Input: part model. Units: mm. Frame: model coordinates. A direction names the side the tool comes from. Give positions to 0.01 mm unless a question says otherwise; leave off trailing zeros. Loops run counter-clockwise (first coordinate to the right, second up) from the corner with the lowest first, then second, coordinate; pieces in that order, holes last. Notation, with made-up numbers: M -32,9.5 L 10,9.5 A8 cw 10,17.5 Z; hole C 62,-17.75 d8. An arc over 180 degrees is marked long. Use CSV: the item, a comma, the result in double quotes. Start each with the question number.
Q1. Reachability of faces 4 (the flat face through (1.2, 4, 1.2)), 5 (the flat face through (4, 7, -10)), 6 (the flat face through (-5.27, 6.93, 6.54)), 7 (the flat face through (-22, 30.5, 0)), 8 (the cylindrical face through (-28.951, 39.495, -0.917)) from +Z, -Z, +X, -X, +Y, -Y: full face, straight path, thin tool, end or side. Return the list, or none.
Q2. Section D-D, the plane z = -12. Output: boundary loops of the cut face in (x, y), plus the area to 3 significant figures.
Q3. Pin query (flat end, axial travel): pin 1 (1 mm diameter, centred on x = -25.5, y = 31.5, fed in from -Z); pin 2 (4 mm diameter, centred on x = 3.5, y = 6, fed in from +Z); pin 3 (1.2 mm diameter, centred on y = 57.5, z = 5, fed in from -X); pin 4 (2 mm diameter, centred on x = -22.5, y = 24.5, fed in from +Z). Return the tip coordinate at first contact, or that it passes through.
Q4. Material intervals for line 1 along Y through (x, z) = (4, 5); line 2 along Y through (x, z) = (1.9, 5); line 3 along Z through (x, y) = (2.95, 57.5), sorted ascending.
Q5. Section C-C, the plane x = -28.5. Output: boundary loops of the cut face in (y, z), plus the area to 3 significant figures.
Q6. Pull-direction query (Y, two-part tool) for faces 1 (the flat face through (-20, 37, 9)), 2 (the cylindrical face through (3.51, 58.34, -5.54)), 3 (the flat face through (-14, 57, 6)); classes: released by +Y, released by -Y, zero draft, split by the parting line, or undercut.
Q7. Section B-B, the plane y = 40.5. Output: boundary loops of the cut face in (x, z) (3 decimals), plus the area to 3 significant figures.
Q8. Section A-A, the plane x = 5. Output: boundary loops of the cut face in (y, z).
from build123d import *

# Parameters (mm, degrees)
SKETCH1_W                  = 40
SKETCH1_H                  = 25
BOSS_EXTRUDE1_DEPTH        = 2
SKETCH2_W                  = 5
SKETCH2_H                  = 20
BOSS_EXTRUDE2_DEPTH        = 10
SKETCH4_W                  = 19.965035534
SKETCH4_H                  = 6
BOSS_EXTRUDE3_DEPTH        = 5
SKETCH5_R                  = 1
CUT_EXTRUDE2_DEPTH         = 5
SKETCH6_W                  = 4
SKETCH6_H                  = 5
BOSS_EXTRUDE4_DEPTH        = 10
SKETCH8_W                  = 5
SKETCH8_H                  = 4
BOSS_EXTRUDE5_DEPTH        = 10
SKETCH9_W                  = 4
SKETCH9_H                  = 5
BOSS_EXTRUDE6_DEPTH        = 45
SKETCH12_W                 = 18
SKETCH12_H                 = 4
BOSS_EXTRUDE8_DEPTH        = 4
SKETCH13_W                 = 5
SKETCH13_H                 = 4
BOSS_EXTRUDE9_DEPTH        = 26
SKETCH14_W                 = 18
SKETCH14_H                 = 4
BOSS_EXTRUDE10_DEPTH       = 6
SKETCH16_W                 = 5.988277512
SKETCH16_H                 = 18
BOSS_EXTRUDE11_DEPTH       = 5
SKETCH15_R                 = 1
CUT_EXTRUDE3_DEPTH         = 6
SKETCH17_R                 = 3
CUT_EXTRUDE5_DEPTH         = 6
SKETCH24_W                 = 8
SKETCH24_H                 = 18.5
BOSS_EXTRUDE18_DEPTH       = 4
BOSS_EXTRUDE20_START       = -1
SKETCH20_R                 = 5
SKETCH20_R_2               = 3
BOSS_EXTRUDE20_DEPTH       = 1
BOSS_EXTRUDE21_OUTLINE_R   = 2.998308623
BOSS_EXTRUDE21_OUTLINE_R_2 = 1.5
BOSS_EXTRUDE21_DEPTH       = 1
SKETCH27_R                 = 5
SKETCH27_R_2               = 2.75
BOSS_EXTRUDE22_DEPTH       = 2
SKETCH28_R                 = 2.75
CUT_EXTRUDE10_DEPTH        = 10
SKETCH31_R                 = 4
BOSS_EXTRUDE23_DEPTH       = 11
SKETCH32_R                 = 23.58495283
BOSS_EXTRUDE24_DEPTH       = 2
SKETCH33_R                 = 3
CUT_EXTRUDE11_DEPTH        = 3
CUT_EXTRUDE12_DEPTH        = 10
CUT_EXTRUDE13_DEPTH        = 4
BOSS_EXTRUDE25_DEPTH       = 2
CUT_EXTRUDE15_DEPTH        = 2
SKETCH38_W                 = 4
SKETCH38_H                 = 6
CUT_EXTRUDE16_DEPTH        = 76.679363321
BOSS_EXTRUDE26_DEPTH       = 5


# Read off the part's stored shape, not the designer's step: Boss-Extrude21
with BuildPart() as part:
    # Sketch1 → Boss-Extrude1 (new body)
    with BuildSketch(Plane(origin=(0, 0, 0), x_dir=(1, 0, 0), z_dir=(0, 1, 0))):
        Rectangle(SKETCH1_W, SKETCH1_H)
    extrude(amount=BOSS_EXTRUDE1_DEPTH)

    # Sketch2 → Boss-Extrude2 (add)
    with BuildSketch(Plane(origin=(0, 2, 0), x_dir=(1, 0, 0), z_dir=(0, 1, 0))):
        with Locations((4.5, 0)):
            Rectangle(SKETCH2_W, SKETCH2_H)
    extrude(amount=BOSS_EXTRUDE2_DEPTH)

    # Sketch4 → Boss-Extrude3 (add)
    with BuildSketch(Plane(origin=(7, 0, 0), x_dir=(0, 0, -1), z_dir=(1, 0, 0))):
        with Locations((-0.017482233, 9)):
            Rectangle(SKETCH4_W, SKETCH4_H)
    extrude(amount=-BOSS_EXTRUDE3_DEPTH)

    # Sketch5 → Cut-Extrude2 (cut)
    with BuildSketch(Plane(origin=(7, 0, 0), x_dir=(0, 0, -1), z_dir=(1, 0, 0))):
        with Locations((5, 7.5)):
            Circle(SKETCH5_R)
        with Locations((-5, 7.5)):
            Circle(SKETCH5_R)
    extrude(amount=-CUT_EXTRUDE2_DEPTH, mode=Mode.SUBTRACT)

    # Sketch6 → Boss-Extrude4 (add)
    with BuildSketch(Plane(origin=(0, 2, 0), x_dir=(1, 0, 0), z_dir=(0, 1, 0))):
        with Locations((-11.527661753, -6.5)):
            Rectangle(SKETCH6_W, SKETCH6_H)
        with Locations((-11.527661753, 6.5)):
            Rectangle(SKETCH6_W, SKETCH6_H)
    extrude(amount=BOSS_EXTRUDE4_DEPTH)

    # Sketch8 → Boss-Extrude5 (add)
    with BuildSketch(Plane.ZY.offset(13.527661753)):
        with Locations((-6.5, 10)):
            Rectangle(SKETCH8_W, SKETCH8_H)
    boss_extrude5 = extrude(amount=BOSS_EXTRUDE5_DEPTH)

    # Mirror1: Boss-Extrude5 across plane
    add(boss_extrude5.mirror(Plane(origin=(0, 0, 0), x_dir=(1, 0, 0), z_dir=(0, 0, -1))))

    # Sketch9 → Boss-Extrude6 (add)
    with BuildSketch(Plane(origin=(0, 12, 0), x_dir=(1, 0, 0), z_dir=(0, 1, 0))):
        with Locations((-21.527661753, 6.5)):
            Rectangle(SKETCH9_W, SKETCH9_H)
    boss_extrude6 = extrude(amount=BOSS_EXTRUDE6_DEPTH)

    # Mirror2: Boss-Extrude5 across plane
    add(boss_extrude5.mirror(Plane(origin=(0, 0, 0), x_dir=(1, 0, 0), z_dir=(0, 0, -1))))

    # Mirror3: Boss-Extrude6 across plane
    add(boss_extrude6.mirror(Plane(origin=(0, 0, 0), x_dir=(1, 0, 0), z_dir=(0, 0, -1))))

    # Sketch12 → Boss-Extrude8 (add)
    with BuildSketch(Plane.ZY.offset(23.527661753)):
        with Locations((0, 55)):
            Rectangle(SKETCH12_W, SKETCH12_H)
        with Locations((0, 10)):
            Rectangle(SKETCH12_W, SKETCH12_H)
        with Locations((0, 32.5)):
            Rectangle(SKETCH12_W, SKETCH12_H)
    extrude(amount=-BOSS_EXTRUDE8_DEPTH)

    # Sketch13 → Boss-Extrude9 (add)
    with BuildSketch(Plane(origin=(-19.527661753, 0, 0), x_dir=(0, 0, -1), z_dir=(1, 0, 0))):
        with Locations((-6.5, 55)):
            Rectangle(SKETCH13_W, SKETCH13_H)
        with Locations((6.5, 55)):
            Rectangle(SKETCH13_W, SKETCH13_H)
    extrude(amount=BOSS_EXTRUDE9_DEPTH)

    # Sketch14 → Boss-Extrude10 (add)
    with BuildSketch(Plane(origin=(6.472338247, 0, 0), x_dir=(0, 0, -1), z_dir=(1, 0, 0))):
        with Locations((0, 55)):
            Rectangle(SKETCH14_W, SKETCH14_H)
    extrude(amount=-BOSS_EXTRUDE10_DEPTH)

    # Sketch16 → Boss-Extrude11 (add)
    with BuildSketch(Plane(origin=(0, 57, 0), x_dir=(1, 0, 0), z_dir=(0, 1, 0))):
        with Locations((3.478199491, 0)):
            Rectangle(SKETCH16_W, SKETCH16_H)
    extrude(amount=BOSS_EXTRUDE11_DEPTH)

    # Sketch15 → Cut-Extrude3 (cut)
    with BuildSketch(Plane(origin=(6.472338247, 0, 0), x_dir=(0, 0, -1), z_dir=(1, 0, 0))):
        with Locations((-5, 57.5)):
            Circle(SKETCH15_R)
        with Locations((5, 57.5)):
            Circle(SKETCH15_R)
    extrude(amount=-CUT_EXTRUDE3_DEPTH, mode=Mode.SUBTRACT)

    # Sketch17 → Cut-Extrude5 (cut)
    with BuildSketch(Plane.XZ):
        with Locations(Location((0, 0, 0), (0, 0, 270))):
            Circle(SKETCH17_R)
    extrude(amount=-CUT_EXTRUDE5_DEPTH, mode=Mode.SUBTRACT)

    # Sketch24 → Boss-Extrude18 (add)
    with BuildSketch(Plane.ZY.offset(23.527661753)):
        with Locations((0, 43.75)):
            Rectangle(SKETCH24_W, SKETCH24_H)
    extrude(amount=-BOSS_EXTRUDE18_DEPTH)

    # Sketch20 → Boss-Extrude20 (add)
    with BuildSketch(Plane(origin=(0, 3, 0), x_dir=(1, 0, 0), z_dir=(0, 1, 0)).offset(BOSS_EXTRUDE20_START)):
        Circle(SKETCH20_R)
        with Locations(Location((0, 0, 0), (0, 0, 90))):
            Circle(SKETCH20_R_2, mode=Mode.SUBTRACT)
    extrude(amount=BOSS_EXTRUDE20_DEPTH)

    # Boss-Extrude21 outline → Boss-Extrude21 (add)
    # profile 1 of 2: a face of its own
    with BuildSketch(Plane(origin=(0, 3, 0), x_dir=(1, 0, 0), z_dir=(0, 1, 0))):
        with BuildLine():
            ThreePointArc((2, -2.236067977), (-3, 0), (2, 2.236067977))
            Line((2, 2.236067977), (2, 4.582575695))
            ThreePointArc((2, 4.582575695), (-5, 0), (2, -4.582575695))
            Line((2, -4.582575695), (2, -2.236067977))
        make_face()
    # profile 2 of 2: a face of its own
    with BuildSketch(Plane(origin=(0, 3, 0), x_dir=(1, 0, 0), z_dir=(0, 1, 0))):
        Circle(BOSS_EXTRUDE21_OUTLINE_R)
        Circle(BOSS_EXTRUDE21_OUTLINE_R_2, mode=Mode.SUBTRACT)
    extrude(amount=BOSS_EXTRUDE21_DEPTH)

    # Sketch27 → Boss-Extrude22 (add)
    with BuildSketch(Plane(origin=(0, 4, 0), x_dir=(1, 0, 0), z_dir=(0, 1, 0))):
        Circle(SKETCH27_R)
        with Locations(Location((0, 0, 0), (0, 0, 43.341758227))):
            Circle(SKETCH27_R_2, mode=Mode.SUBTRACT)
    extrude(amount=BOSS_EXTRUDE22_DEPTH)

    # Sketch28 → Cut-Extrude10 (cut)
    with BuildSketch(Plane(origin=(0, 6, 0), x_dir=(1, 0, 0), z_dir=(0, 1, 0))):
        with Locations(Location((0, 0, 0), (0, 0, 43.341758227))):
            Circle(SKETCH28_R)
    extrude(amount=CUT_EXTRUDE10_DEPTH, mode=Mode.SUBTRACT)

    # Sketch31 → Boss-Extrude23 (add)
    with BuildSketch(Plane.ZY.offset(23.527661753)):
        with Locations((-0.05, 43.4)):
            Circle(SKETCH31_R)
    extrude(amount=BOSS_EXTRUDE23_DEPTH)

    # Sketch32 → Boss-Extrude24 (add)
    with BuildSketch(Plane.XZ):
        with Locations(Location((0, 0, 0), (0, 0, 270))):
            Circle(SKETCH32_R)
    extrude(amount=-BOSS_EXTRUDE24_DEPTH)

    # Sketch33 → Cut-Extrude11 (cut)
    with BuildSketch(Plane.XZ):
        with Locations(Location((0, 0, 0), (0, 0, 270))):
            Circle(SKETCH33_R)
    extrude(amount=-CUT_EXTRUDE11_DEPTH, mode=Mode.SUBTRACT)

    # Sketch34 → Cut-Extrude12 (cut)
    with BuildSketch(Plane(origin=(0, 2, 0), x_dir=(1, 0, 0), z_dir=(0, 1, 0))):
        with BuildLine():
            Line((-10.212765957, 21.718642027), (-10.212765957, 13.952471709))
            Line((-10.212765957, 13.952471709), (10.212765957, 13.952471709))
            Line((10.212765957, 13.952471709), (10.212765957, 21.718642027))
            ThreePointArc((10.212765957, 21.718642027), (0, 24), (-10.212765957, 21.718642027))
        make_face()
    extrude(amount=-CUT_EXTRUDE12_DEPTH, mode=Mode.SUBTRACT)

    # Sketch35 → Cut-Extrude13 (cut)
    with BuildSketch(Plane.XZ):
        with BuildLine():
            Line((-17.290808405, 0), (-23.58495283, 0))
            ThreePointArc((-23.58495283, 0), (-19.96393753, -12.557515611), (-10.212765957, -21.259101851))
            Line((-10.212765957, -21.259101851), (-10.212765957, -13.952471709))
            ThreePointArc((-10.212765957, -13.952471709), (-15.420101082, -7.822565942), (-17.290808405, 0))
        make_face()
    extrude(amount=-CUT_EXTRUDE13_DEPTH, mode=Mode.SUBTRACT)

    # Sketch36 → Boss-Extrude25 (add)
    with BuildSketch(Plane.XZ):
        with BuildLine():
            Line((-10.212765957, -13.952471709), (10.212765957, -13.952471709))
            ThreePointArc((10.212765957, -13.952471709), (0, -17.290808405), (-10.212765957, -13.952471709))
        make_face()
    extrude(amount=-BOSS_EXTRUDE25_DEPTH)

    # Sketch37 → Cut-Extrude15 (cut)
    with BuildSketch(Plane.XZ):
        with BuildLine():
            Line((-23.58495283, 0), (-17.290808405, 0))
            ThreePointArc((-17.290808405, 0), (7.822565942, 15.420101082), (10.212765957, -13.952471709))
            Line((10.212765957, -13.952471709), (10.212765957, -21.259101851))
            ThreePointArc((10.212765957, -21.259101851), (12.557515611, 19.96393753), (-23.58495283, 0))
        make_face()
    extrude(amount=-CUT_EXTRUDE15_DEPTH, mode=Mode.SUBTRACT)

    # Sketch38 → Cut-Extrude16 (cut, through all)
    with BuildSketch(Plane.XY.offset(9)):
        with Locations((-11.527661753, 5)):
            Rectangle(SKETCH38_W, SKETCH38_H)
    extrude(amount=-CUT_EXTRUDE16_DEPTH, mode=Mode.SUBTRACT)


with BuildPart() as cut_extrude16_piece_1:
    # of the separate pieces the step leaves, piece 1, a body of its own (cut_extrude16_pieces)
    add(part.part.solids().sort_by_distance((-9.527661753, 8, -4))[0])



with BuildPart() as cut_extrude16_piece_2:
    # of the separate pieces the step leaves, piece 2, a body of its own (cut_extrude16_pieces)
    add(part.part.solids().sort_by_distance((-17.290808405, 0, 0))[0])


with BuildPart() as cut_extrude16_piece_1_1:
    add(cut_extrude16_piece_1.part)

    add(cut_extrude16_piece_2.part)  # Boss-Extrude26 merges Cut-Extrude16 piece 2
    # Sketch39 → Boss-Extrude26 (add)
    with BuildSketch(Plane.XY.offset(9)):
        Polygon((-9.527661753, 8), (-8.439950649, 2), (-4.374753349, 2), (-6.187605188, 12), (-9.527661753, 12), align=None)
    boss_extrude26 = extrude(amount=-BOSS_EXTRUDE26_DEPTH)

    # Mirror4: Boss-Extrude26 across plane
    add(boss_extrude26.mirror(Plane(origin=(0, 0, 0), x_dir=(1, 0, 0), z_dir=(0, 0, -1))))


solid = cut_extrude16_piece_1_1.part
A:
1,face 4,"none"
1,face 5,"-Z, +X, -X, +Y"
1,face 6,"+Z"
1,face 7,"+X, -X"
1,face 8,"-X"
2,outline,"M -12.45,0 L 12.45,0 L 12.45,2 L -12.45,2 Z"
2,area,"49.8 mm^2"
3,pin 1,"through"
3,pin 2,"z = 10"
3,pin 3,"x = -23.53"
3,pin 4,"z = 9"
4,line 1,"0 to 6.5, 8.5 to 12, 53 to 56.5, 58.5 to 62"
4,line 2,"0 to 2, 53 to 56.5, 58.5 to 62"
4,line 3,"-9 to -6, -4 to 4, 6 to 9"
5,outline,"C 43.4,-0.05 d8"
5,area,"50.3 mm^2"
6,face 1,"zero draft"
6,face 2,"undercut"
6,face 3,"released by +Y"
7,outline,"M -34.528,-2.805 L -23.528,-2.805 L -23.528,-9 L -19.528,-9 L -19.528,9 L -23.528,9 L -23.528,2.705 L -34.528,2.705 Z"
7,area,"133 mm^2"
8,outline,"M 0,-16.55 L 2,-16.55 L 2,-10 L 12,-10 L 12,10 L 2,10 L 2,16.55 L 0,16.55 Z; M 53,-9 L 62,-9 L 62,9 L 53,9 Z; hole C 7.5,-5 d2; hole C 7.5,5 d2; hole C 57.5,-5 d2; hole C 57.5,5 d2"
